Read the model definition and answer for the solid it produces. Units are mm, in the model's axes. A direction names the side the tool comes from. Coordinates: 2 decimals unless noted, no trailing zeros. Order: outer loops, then holes, each group sorted by start corner. A loop starts at its lowest first (then second) coordinate and runs counter-clockwise, first axis right, second up. Notation, with made-up numbers: (8, 39.25) -> (54, 39.25) arc R17 cw to (54, 69.25) -> close; hole circle Ø4 at (70.5, 60.25). An arc over 180 degrees is marked (long way). Answer as a JSON object with one key per item and string values. Group by question number.
1) Given pin 1 (5 mm diameter, centred on y = 18.5, z = 15, fed in from -X); pin 2 (5 mm diameter, centred on x = 19.5, z = 17.5, fed in from +Y); pin 3 (5 mm diameter, centred on y = 10.5, z = 14, fed in from +X), each flat-ended and moving along its own axis, determine where each tip first touches the part or whether it passes through.
2) Section A-A on z = 11 is taken. Determine the outline of the cut face in (x, y).
3) A tool of negligible diameter and unlimited length cuts with its end or side. For faces 5 (the cylindrical face through (34.278, 0.684, 1.521)), 6 (the cylindrical face through (22.923, 18.302, 16.345)), from which of +Z, -Z, +X, -X, +Y, -Y can it reach the whole face along a straight path? Write none if from no direction.
4) Consider L1, parallel to Z at x = 10, y = 10.5; L2, parallel to Z at x = 18, y = 13; L3, parallel to Z at x = 20, y = 13.5. Determine where each line is inside the solid, lowest interval first.
5) Determine the mould class of faces 1 (the flat face through (17, 15, 0)), 2 (the flat face through (13, 9, 3)), 3 (the cylindrical face through (16.013, 16.637, 25.867)), 4 (the flat face through (35, 15, 1)) for opening direction Z: released by +Z, released by -Z, zero draft, split by the parting line, or undercut.
6) Section B-B on y = 3.5 is taken. Determine the outline of the cut face in (x, z), and give its area (3 significant figures).
from build123d import *

# Parameters (mm, degrees)
CYLINDER001_R               = 2
CYLINDER001_DEPTH           = 25
CYLINDER001_PLACEMENT_ANGLE = 101.1
BOX_W                       = 35
BOX_H                       = 30
BOX_DEPTH                   = 3
CYLINDER_R                  = 6
CYLINDER_DEPTH              = 30
FILLET_R                    = 2.4
FILLET001_R                 = 2.4


with BuildPart() as cylinder001:
    # Cylinder001 → Cylinder001 (new body)
    with BuildSketch(Plane.XY):
        Circle(CYLINDER001_R)
    extrude(amount=CYLINDER001_DEPTH)


with BuildPart() as cylinder001_1:
    # Cylinder001 placement: moved
    add(cylinder001.part.moved(Location((17.6, 6.769902, 26.562882))).rotate(Axis((17.6, 6.769902, 26.562882), (-1, 0, 0)), CYLINDER001_PLACEMENT_ANGLE))


with BuildPart() as box:
    # Box → Box (new body)
    with BuildSketch(Plane.XY):
        with Locations((17.5, 15)):
            Rectangle(BOX_W, BOX_H)
    extrude(amount=BOX_DEPTH)


with BuildPart() as fillet001:
    # Cylinder → Cylinder (new body)
    with BuildSketch(Plane(origin=(17.2, 16.5, 0), x_dir=(1, 0, 0), z_dir=(0, 0, 1))):
        Circle(CYLINDER_R)
    extrude(amount=CYLINDER_DEPTH)

    # Fusion: union Box
    add(box.part)

    # Cut: cut Cylinder001
    add(cylinder001_1.part, mode=Mode.SUBTRACT)

    # Fillet
    fillet_edges = [fillet001.edges().sort_by_distance(p)[0] for p in [
        (11.2, 16.5, 3),
    ]]
    fillet(fillet_edges, radius=FILLET_R)

    # Fillet001
    fillet001_edges = [fillet001.edges().sort_by_distance(p)[0] for p in [
        (11.2, 16.5, 30),
        (0, 0, 1.5),
        (0, 30, 1.5),
        (35, 30, 1.5),
        (35, 0, 1.5),
    ]]
    fillet(fillet001_edges, radius=FILLET001_R)


solid = fillet001.part
Worked answers:
{
 "1": {"pin 1": "stops at x = 11.2", "pin 2": "stops at y = 22.5", "pin 3": "stops at x = 22.07"},
 "2": {"outline": "circle Ø12 at (17.2, 16.5)"},
 "3": {"face 5": "+Z, -Z, +X, -Y", "face 6": "+Z"},
 "4": {"L1": "z = 0 to 3", "L2": "z = 0 to 23.34, 27.34 to 30", "L3": "z = 0 to 29.95"},
 "5": {"face 1": "released by -Z", "face 2": "released by +Z", "face 3": "undercut", "face 4": "zero draft"},
 "6": {"outline": "(0, 0) -> (35, 0) -> (35, 3) -> (0, 3) -> close", "area": "105 mm²"}
}
